from build123d import *

# Parameters (mm, degrees)
SKETCH1_R                                           = 70
SKETCH1_R_2                                         = 45
BOSS_EXTRUDE1_DEPTH                                 = 4
SKETCH2_R                                           = 53
SKETCH2_R_2                                         = 45
BOSS_EXTRUDE2_DEPTH                                 = 53
SKETCH4_W                                           = 13.25
SKETCH4_H                                           = 8
SKETCH4_W_2                                         = 8
SKETCH4_H_2                                         = 39
BOSS_EXTRUDE4_DEPTH                                 = 13
BOSS_EXTRUDE5_DEPTH                                 = 4
SKETCH7_R                                           = 1.3
CUT_EXTRUDE4_DEPTH                                  = 7.2
SKETCH9_W                                           = 10
SKETCH9_H                                           = 25
CUT_EXTRUDE7_DEPTH                                  = 8
CUT_EXTRUDE9_DEPTH                                  = 113.289803633
CSK_FOR_M3_COUNTERSUNK_FLAT_HEAD_SCREW1_D           = 3.4
CSK_FOR_M3_COUNTERSUNK_FLAT_HEAD_SCREW1_CSINK_D     = 6.3
CSK_FOR_M3_COUNTERSUNK_FLAT_HEAD_SCREW1_CSINK_ANGLE = 90
SKETCH18_R                                          = 53
SKETCH18_R_2                                        = 48.6
BOSS_EXTRUDE6_DEPTH                                 = 5
CUT_EXTRUDE10_DEPTH                                 = 1


with BuildPart() as part:
    # Sketch1 → Boss-Extrude1 (new body)
    with BuildSketch(Plane(origin=(0, 0, 0), x_dir=(1, 0, 0), z_dir=(0, 1, 0))):
        with Locations(Location((0, 0, 0), (0, 0, 270))):
            Circle(SKETCH1_R)
        with Locations(Location((0, 0, 0), (0, 0, 270))):
            Circle(SKETCH1_R_2, mode=Mode.SUBTRACT)
    extrude(amount=BOSS_EXTRUDE1_DEPTH)

    # Sketch2 → Boss-Extrude2 (add)
    with BuildSketch(Plane(origin=(0, 4, 0), x_dir=(1, 0, 0), z_dir=(0, 1, 0))):
        with Locations(Location((0, 0, 0), (0, 0, 270))):
            Circle(SKETCH2_R)
        with Locations(Location((0, 0, 0), (0, 0, 270))):
            Circle(SKETCH2_R_2, mode=Mode.SUBTRACT)
    extrude(amount=BOSS_EXTRUDE2_DEPTH)

    # Sketch4 → Boss-Extrude4 (add, symmetric)
    with BuildSketch(Plane.XY):
        with Locations((-38.375, 35)):
            Rectangle(SKETCH4_W, SKETCH4_H)
        Polygon((-31.75, 31), (-45, 31), (-45, 17.75), align=None)
        with Locations((15.25, 19.5)):
            Rectangle(SKETCH4_W_2, SKETCH4_H_2)
    extrude(amount=BOSS_EXTRUDE4_DEPTH, both=True)


with BuildPart() as boss_extrude4_piece_1:
    # of the separate pieces the step leaves, piece 1, a body of its own (boss_extrude4_pieces)
    add(part.part.solids().sort_by_distance((0, 0, 70))[0])



with BuildPart() as boss_extrude4_piece_2:
    # of the separate pieces the step leaves, piece 2, a body of its own (boss_extrude4_pieces)
    add(part.part.solids().sort_by_distance((11.25, 39, -13))[0])


with BuildPart() as boss_extrude4_piece_1_1:
    add(boss_extrude4_piece_1.part)

    add(boss_extrude4_piece_2.part)  # Boss-Extrude5 merges Boss-Extrude4 piece 2
    # Sketch5 → Boss-Extrude5 (add)
    with BuildSketch(Plane.XZ):
        with BuildLine():
            Line((11.25, 13), (29.067400866, 34.352382842))
            ThreePointArc((29.067400866, 34.352382842), (45, 0), (29.067400866, -34.352382842))
            Line((29.067400866, -34.352382842), (11.25, -13))
            Line((11.25, -13), (11.25, 13))
        make_face()
    extrude(amount=-BOSS_EXTRUDE5_DEPTH)

    # Sketch7 → Cut-Extrude4 (cut)
    with BuildSketch(Plane(origin=(0, 39, 0), x_dir=(1, 0, 0), z_dir=(0, 1, 0))):
        with Locations(Location((-34.25, 5, 0), (0, 0, 180))):
            Circle(SKETCH7_R)
        with Locations(Location((-34.25, -5, 0), (0, 0, 180))):
            Circle(SKETCH7_R)
        with Locations(Location((13.75, 5, 0), (0, 0, 180))):
            Circle(SKETCH7_R)
        with Locations(Location((13.75, -5, 0), (0, 0, 180))):
            Circle(SKETCH7_R)
    extrude(amount=-CUT_EXTRUDE4_DEPTH, mode=Mode.SUBTRACT)

    # Sketch9 → Cut-Extrude7 (cut)
    with BuildSketch(Plane.ZY.offset(-11.25)):
        with Locations((0, 17.5)):
            Rectangle(SKETCH9_W, SKETCH9_H)
    extrude(amount=-CUT_EXTRUDE7_DEPTH, mode=Mode.SUBTRACT)

    # Sketch12 → Cut-Extrude9 (cut, through all)
    with BuildSketch(Plane(origin=(0, 4, 0), x_dir=(1, 0, 0), z_dir=(0, 1, 0))):
        with BuildLine():
            Line((29.479537487, 22.359715328), (27.25, 19.687836398))
            Line((27.25, 19.687836398), (27.25, -19.687836398))
            Line((27.25, -19.687836398), (29.479537487, -22.359715328))
            ThreePointArc((29.479537487, -22.359715328), (37, 0), (29.479537487, 22.359715328))
        make_face()
        Polygon((27.25, -19.687836398), (27.25, 19.687836398), (24.25, 16.092634774), (24.25, -16.092634774), align=None)
    extrude(amount=-CUT_EXTRUDE9_DEPTH, mode=Mode.SUBTRACT)

    # CSK for M3 Countersunk Flat Head Screw1 (through all)
    with Locations(Plane(origin=(0, 4, 0), x_dir=(1, 0, 0), z_dir=(0, 1, 0))):
        with Locations((-43.840620434, 43.840620434), (-43.840620434, -43.840620434), (43.840620434, -43.840620434), (43.840620434, 43.840620434)):
            CounterSinkHole(CSK_FOR_M3_COUNTERSUNK_FLAT_HEAD_SCREW1_D / 2, CSK_FOR_M3_COUNTERSUNK_FLAT_HEAD_SCREW1_CSINK_D / 2, counter_sink_angle=CSK_FOR_M3_COUNTERSUNK_FLAT_HEAD_SCREW1_CSINK_ANGLE)

    # Sketch18 → Boss-Extrude6 (add)
    with BuildSketch(Plane(origin=(0, 57, 0), x_dir=(1, 0, 0), z_dir=(0, 1, 0))):
        with Locations(Location((0, 0, 0), (0, 0, 270))):
            Circle(SKETCH18_R)
        with Locations(Location((0, 0, 0), (0, 0, 270))):
            Circle(SKETCH18_R_2, mode=Mode.SUBTRACT)
    extrude(amount=BOSS_EXTRUDE6_DEPTH)

    # Sketch19 → Cut-Extrude10 (cut, symmetric)
    with BuildSketch(Plane.XY):
        Polygon((-39.75, 39), (-31.75, 36), (-31.75, 39), align=None)
        Polygon((11.25, 39), (19.25, 39), (11.25, 36), align=None)
    extrude(amount=CUT_EXTRUDE10_DEPTH, both=True, mode=Mode.SUBTRACT)


solid = boss_extrude4_piece_1_1.part
Can you work these out from the model? Positions are in its coordinate system, mm. A direction names the side the tool comes from. Round coordinates to 2 decimals unless told otherwise and drop trailing zeros. Loops run counter-clockwise (first coordinate to the right, second up) from the corner with the lowest first, then second, coordinate; pieces in that order, holes last. Notation, with made-up numbers: (31, 63) - (57, 63) arc R20 ccw to (57, 101) - close; hole circle Ø2 at (-3, -31). An arc over 180 degrees is marked (long way). Answer in a Markdown table with one row per item. Add a question column.
Q1. I want a section at D-D on x = -50.5. List the corners of the cut face in (y, z) for me.
Q2. Which directions (+Z, -Z, +X, -X, +Y, -Y) give clear straight access to the entire face, cutting with the end or side of a thin tool? Please do faces 3 (the flat face through (15, 17, -5)), 4 (the flat face through (15, 39, -7)), 5 (the flat face through (24.25, 2, 0)).
Q3. For pin 1 Ø4 at (x, z) = (15, 1) entering from +Y; pin 2 Ø0.9 at (x, y) = (17, 38) entering from -Z; pin 3 Ø10 at (x, y) = (-20.5, 52) entering from +Z, each with a flat end and sliding along its axis, tell me the tip position at first contact or that it passes through.
Q4. I want a section at C-C on y = 22.5. List the corners of the cut face in (x, z) for me.
Q5. We'd pull the mould along X, two halves only. Please class faces 1 (the cylindrical face through (-42.594, 1.972, -55.55)), 2 (the flat face through (11.25, 19, 6)): pulls with the +X half, pulls with the -X half, needs draft (parallel to the pull), parting line crosses it, or undercut.
Q6. I want a section at B-B on x = 0. List the corners of the cut face in (y, z) for me.
Q7. I want a section at A-A on y = 9.5. List the corners of the cut face in (x, z) for me, and give its area (3 significant figures).
Q8. I need wall thicknesses on L1, parallel to X at y = 12.5, z = 11.5; L2, parallel to X at y = 55.5, z = 0; L3, parallel to Z at x = -34.25, y = 34.75. Which ranges of each line are inside material? Lowest first, please.
A:
| question | item | result |
|---|---|---|
| 1 | outline | (0, -48.47) - (4, -48.47) - (4, -16.09) - (62, -16.09) - (62, 16.09) - (4, 16.09) - (4, 48.47) - (0, 48.47) - close |
| 2 | face 3 | none |
| 2 | face 4 | +Y |
| 2 | face 5 | +Y, -Y |
| 3 | pin 1 | y = 39 |
| 3 | pin 2 | z = -50.35 |
| 3 | pin 3 | z = 50.68 |
| 4 | outline | circle Ø106 at (0, 0); (11.25, -13) - (19.25, -13) - (19.25, -5) - (11.25, -5) - close; (11.25, 5) - (19.25, 5) - (19.25, 13) - (11.25, 13) - close; hole (-43.08, -13) arc R45 ccw (long way) to (-43.08, 13) - (-40.25, 13) - (-40.25, -13) - close |
| 5 | face 1 | parting line crosses it |
| 5 | face 2 | undercut |
| 6 | outline | (0, -70) - (4, -70) - (4, -53) - (62, -53) - (62, -48.6) - (57, -48.6) - (57, -45) - (0, -45) - close; (0, 45) - (57, 45) - (57, 48.6) - (62, 48.6) - (62, 53) - (4, 53) - (4, 70) - (0, 70) - close |
| 7 | outline | circle Ø106 at (0, 0); (11.25, -13) - (19.25, -13) - (19.25, -5) - (11.25, -5) - close; (11.25, 5) - (19.25, 5) - (19.25, 13) - (11.25, 13) - close; hole circle Ø90 at (0, 0) |
| 7 | area | 2,590 mm^2 |
| 8 | L1 | -51.74 to -43.51, 11.25 to 19.25, 43.51 to 51.74 |
| 8 | L2 | -53 to -45, 45 to 53 |
| 8 | L3 | -40.45 to -29.19, -13 to -6.3, -3.7 to 3.7, 6.3 to 13, 29.19 to 40.45 |
